For this review, take the finished solid that the model builds, in its own axes (mm). Round coordinates to 2 decimals unless told otherwise and drop trailing zeros. Order: outer loops, then holes, each group sorted by start corner. A loop starts at its lowest first (then second) coordinate and runs counter-clockwise, first axis right, second up.
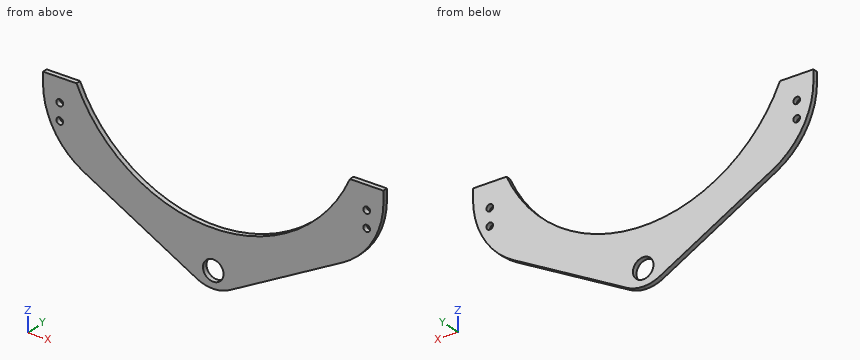
from build123d import *

# Parameters (mm, degrees)
SKETCH1_R           = 4.6
SKETCH1_R_2         = 1.5
BOSS_EXTRUDE2_DEPTH = 3.175
SKETCH2_W           = 235.965281387
SKETCH2_H           = 118.721671229
CUT_EXTRUDE1_DEPTH  = 1.016


with BuildPart() as part:
    # Sketch1 → Boss-Extrude2 (new body)
    with BuildSketch(Plane(origin=(0, 0, 0), x_dir=(1, 0, 0), z_dir=(0, 1, 0))):
        with BuildLine():
            Line((-7.5, 0), (0, 0))
            ThreePointArc((0, 0), (61.2, 39.907584028), (122.4, 0))
            Line((122.4, 0), (129.9, 0))
            Line((129.9, 0), (137.4, 0))
            Line((137.4, 0), (137.4, 4.627434139))
            ThreePointArc((137.4, 4.627434139), (132.49819386, 22.490768832), (119.165787065, 35.350526172))
            Line((119.165787065, 35.350526172), (68.55887696, 62.967039443))
            ThreePointArc((68.55887696, 62.967039443), (65.081261882, 64.334538033), (61.373539646, 64.8))
            Line((61.373539646, 64.8), (61.026460354, 64.8))
            ThreePointArc((61.026460354, 64.8), (57.318738118, 64.334538033), (53.84112304, 62.967039443))
            Line((53.84112304, 62.967039443), (3.234212935, 35.350526172))
            ThreePointArc((3.234212935, 35.350526172), (-10.09819386, 22.490768832), (-15, 4.627434139))
            Line((-15, 4.627434139), (-15, 0))
            Line((-15, 0), (-7.5, 0))
        make_face()
        with Locations(Location((61.2, 57.3, 0), (0, 0, 270))):
            Circle(SKETCH1_R, mode=Mode.SUBTRACT)
        with BuildLine():
            ThreePointArc((-7.5, 8.9), (-9, 10.4), (-7.5, 11.9))
            ThreePointArc((-7.5, 11.9), (-6, 10.4), (-7.5, 8.9))
        make_face(mode=Mode.SUBTRACT)
        with Locations(Location((-7.5, 17.9, 0), (0, 0, 270))):
            Circle(SKETCH1_R_2, mode=Mode.SUBTRACT)
        with BuildLine():
            ThreePointArc((129.9, 8.9), (128.4, 10.4), (129.9, 11.9))
            ThreePointArc((129.9, 11.9), (131.4, 10.4), (129.9, 8.9))
        make_face(mode=Mode.SUBTRACT)
        with Locations(Location((129.9, 17.9, 0), (0, 0, 270))):
            Circle(SKETCH1_R_2, mode=Mode.SUBTRACT)
    extrude(amount=BOSS_EXTRUDE2_DEPTH)

    # Sketch2 → Cut-Extrude1 (cut)
    with BuildSketch(Plane(origin=(0, 3.175, 0), x_dir=(1, 0, 0), z_dir=(0, 1, 0))):
        with Locations((50.311488443, 30.817995662)):
            Rectangle(SKETCH2_W, SKETCH2_H)
    extrude(amount=-CUT_EXTRUDE1_DEPTH, mode=Mode.SUBTRACT)


solid = part.part
(1) Add section C-C on z = -10.4. Give the boundary of the cut face in (x, y), plus the area to 3 significant figures.
(2) Add section D-D on x = 129.9. Give the boundary of the cut face in (y, z).
(3) Add section B-B on z = -22.5. Give the boundary of the cut face in (x, y).
(4) Add section A-A on y = 0.75. Give the boundary of the cut face in (x, z), plus the area to 3 significant figures.
(5) Clearance check with flat-ended pins moving along their axes: P1, Ø10.5, axis at x = 61.2, z = -57.3, coming from the +Y side; P2, Ø1, axis at y = 0.5, z = -41, coming from the +X side. State where each tip first meets the part, or that it passes through.
(6) Wall thickness on L1, parallel to Z at x = 129.9, y = 1.4; L2, parallel to X at y = 0.35, z = -17; L3, parallel to X at y = 1.25, z = -10.4: over which ranges is each line inside the solid? List them lowest first.
Here are the results:
1. outline: (-14.52, 0) - (-9, 0) - (-9, 2.16) - (-14.52, 2.16) - close; (-6, 0) - (5.74, 0) - (5.74, 2.16) - (-6, 2.16) - close; (116.66, 0) - (128.4, 0) - (128.4, 2.16) - (116.66, 2.16) - close; (131.4, 0) - (136.92, 0) - (136.92, 2.16) - (131.4, 2.16) - close
1. area: 74.5 mm2
2. outline: (0, -26.28) - (2.16, -26.28) - (2.16, -19.4) - (0, -19.4) - close; (0, -16.4) - (2.16, -16.4) - (2.16, -11.9) - (0, -11.9) - close; (0, -8.9) - (2.16, -8.9) - (2.16, 0) - (0, 0) - close
3. outline: (-10.09, 0) - (16.2, 0) - (16.2, 2.16) - (-10.09, 2.16) - close; (106.2, 0) - (132.49, 0) - (132.49, 2.16) - (106.2, 2.16) - close
4. outline: (-15, -4.63) arc R35 ccw to (3.23, -35.35) - (53.84, -62.97) arc R15 ccw to (61.03, -64.8) - (61.37, -64.8) arc R15 ccw to (68.56, -62.97) - (119.17, -35.35) arc R35 ccw to (137.4, -4.63) - (137.4, 0) - (122.4, 0) arc R66.88 cw to (0, 0) - (-15, 0) - close; hole circle Ø3 at (-7.5, -17.9); hole circle Ø3 at (-7.5, -10.4); hole circle Ø9.2 at (61.2, -57.3); hole circle Ø3 at (129.9, -17.9); hole circle Ø3 at (129.9, -10.4)
4. area: 3,270 mm2
5. P1: stops at y = 2.16
5. P2: stops at x = 109.73
6. L1: z = -26.28 to -19.4, -16.4 to -11.9, -8.9 to 0
6. L2: x = -12.74 to -8.7, -6.3 to 10.81, 111.59 to 128.7, 131.1 to 135.14
6. L3: x = -14.52 to -9, -6 to 5.74, 116.66 to 128.4, 131.4 to 136.92
